Input: part model. Units: mm. Frame: model coordinates. Face numbers are marked on the shaded views. A direction names the side the tool comes from. Round coordinates to 2 decimals unless told otherwise and drop trailing zeros. Loops run counter-clockwise (first coordinate to the right, second up) from the corner with the lowest first, then second, coordinate; pieces in that order, holes last. Notation, with made-up numbers: M -20.5,45.25 L -8.5,45.25 A22 ccw -8.5,65.25 Z; hole C -34,-26.75 d11. An arc over 180 degrees is marked long. Put each result on its own line as item: value. Start each with the question number.
1) Line query: probe 1 along X at (y, z) = (0, 28.5); probe 2 along X at (y, z) = (-14, 17); probe 3 along Y at (x, z) = (20, 1.35). Output: solid intervals per line, ascending.
2) Pin query (flat end, axial travel): pin 1 (17 mm diameter, centred on x = 10, y = 0, fed in from +Z); pin 2 (8 mm diameter, centred on x = -21.5, z = 24, fed in from +Y); pin 3 (2 mm diameter, centred on y = 6.5, z = 20.5, fed in from -X); pin 4 (1 mm diameter, centred on x = 42, y = 0.5, fed in from +Z). Return the tip coordinate at first contact, or that it passes through.
3) Draft query along X for the marked faces 5, 6 and 7. Return one class per face: +X half, -X half, draft (parallel to the pull), parting line (faces both ways), or undercut.
4) Section D-D on y = -8. Output: boundary loops of the cut face in (x, z).
5) Section C-C on y = -14.5. Output: boundary loops of the cut face in (x, z), plus the area to 3 significant figures.
6) Reachability of the marked faces 1, 2, 3 and 4 from +Z, -Z, +X, -X, +Y, -Y: full face, straight path, thin tool, end or side. Return the list, or none.
7) Section B-B on x = 28. Output: boundary loops of the cut face in (y, z).
8) Section A-A on z = 37.5. Output: boundary loops of the cut face in (x, y).
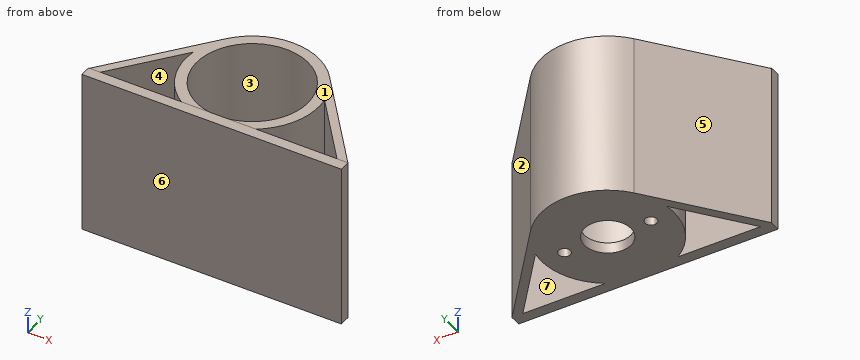
from build123d import *

# Parameters (mm, degrees)
SKETCH1_R           = 30.75
SKETCH1_R_2         = 25.75
BOSS_EXTRUDE2_DEPTH = 76
SKETCH2_R           = 25.75
BOSS_EXTRUDE3_DEPTH = 5
SKETCH3_R           = 10.75
CUT_EXTRUDE1_DEPTH  = 5
SKETCH8_R           = 2.75
CUT_EXTRUDE3_DEPTH  = 5
SKETCH9_W           = 120
SKETCH9_H           = 76.288316085
BOSS_EXTRUDE4_DEPTH = 5
BOSS_EXTRUDE5_DEPTH = 76


with BuildPart() as part:
    # Sketch1 → Boss-Extrude2 (new body)
    with BuildSketch(Plane.XY):
        Circle(SKETCH1_R)
        Circle(SKETCH1_R_2, mode=Mode.SUBTRACT)
    extrude(amount=BOSS_EXTRUDE2_DEPTH)

    # Sketch2 → Boss-Extrude3 (add)
    with BuildSketch(Plane(origin=(0, 0, 0), x_dir=(-1, 0, 0), z_dir=(0, 0, -1))):
        Circle(SKETCH2_R)
    extrude(amount=-BOSS_EXTRUDE3_DEPTH)

    # Sketch3 → Cut-Extrude1 (cut)
    with BuildSketch(Plane(origin=(0, 0, 0), x_dir=(-1, 0, 0), z_dir=(0, 0, -1))):
        Circle(SKETCH3_R)
    extrude(amount=-CUT_EXTRUDE1_DEPTH, mode=Mode.SUBTRACT)

    # Sketch8 → Cut-Extrude3 (cut)
    with BuildSketch(Plane(origin=(0, 0, 0), x_dir=(-1, 0, 0), z_dir=(0, 0, -1))):
        with Locations((20, 0)):
            Circle(SKETCH8_R)
        with Locations(Location((-20, 0, 0), (0, 0, 180))):
            Circle(SKETCH8_R)
    extrude(amount=-CUT_EXTRUDE3_DEPTH, mode=Mode.SUBTRACT)

    # Sketch9 → Boss-Extrude4 (add)
    with BuildSketch(Plane(origin=(0, -30.75, 0), x_dir=(1, 0, 0), z_dir=(0, 1, 0))):
        with Locations((0, -38.144158043)):
            Rectangle(SKETCH9_W, SKETCH9_H)
    extrude(amount=BOSS_EXTRUDE4_DEPTH)

    # Sketch11 → Boss-Extrude5 (add, through all)
    with BuildSketch(Plane.XY.offset(76)):
        Polygon((-60, -25.75), (-24.006301312, 19.21613898), (-30.32899646, 5.070944065), (-55, -25.75), align=None)
        Polygon((55, -25.75), (30.32899646, 5.070944065), (24.006301312, 19.21613898), (60, -25.75), align=None)
    extrude(amount=-BOSS_EXTRUDE5_DEPTH)


solid = part.part
Geometry results:
1. probe 1: x = -39.39 to -34.39, -30.75 to -25.75, 25.75 to 30.75, 34.39 to 39.39
1. probe 2: x = -50.59 to -45.59, -27.38 to -21.61, 21.61 to 27.38, 45.59 to 50.59
1. probe 3: y = -30.75 to -25.75, -23.36 to -2.75, 2.75 to 23.36
2. pin 1: stops at z = 5
2. pin 2: stops at y = 25.28
2. pin 3: stops at x = -34.99
2. pin 4: passes through
3. face 5: -X half
3. face 6: draft
3. face 7: undercut
4. outline: M -45.79,0 L -40.79,0 L -40.79,76 L -45.79,76 Z; M -29.69,0 L -7.18,0 L -7.18,5 L -24.48,5 L -24.48,76 L -29.69,76 Z; M 7.18,0 L 29.69,0 L 29.69,76 L 24.48,76 L 24.48,5 L 7.18,5 Z; M 40.79,0 L 45.79,0 L 45.79,76 L 40.79,76 Z
5. outline: M -50.99,0 L -45.99,0 L -45.99,76 L -50.99,76 Z; M -27.12,0 L 27.12,0 L 27.12,76 L 21.28,76 L 21.28,5 L -21.28,5 L -21.28,76 L -27.12,76 Z; M 45.99,0 L 50.99,0 L 50.99,76 L 45.99,76 Z
5. area: 1,860 mm²
6. face 1: +Z, +X, -X, +Y
6. face 2: +Z, -Z, +X, +Y
6. face 3: +Z
6. face 4: +Z, -Z
7. outline: M -30.75,0 L -25.75,0 L -25.75,76.29 L -30.75,76.29 Z; M -12.71,0 L 14.23,0 L 14.23,76 L -12.71,76 Z
8. outline: M -60,-30.75 L 60,-30.75 L 60,-25.75 L 24.01,19.22 A30.75 ccw -24.01,19.22 L -60,-25.75 Z; hole M -55,-25.75 L -16.81,-25.75 A30.75 cw -30.33,5.07 Z; hole C 0,0 d51.5; hole M 16.81,-25.75 L 55,-25.75 L 30.33,5.07 A30.75 cw Z
